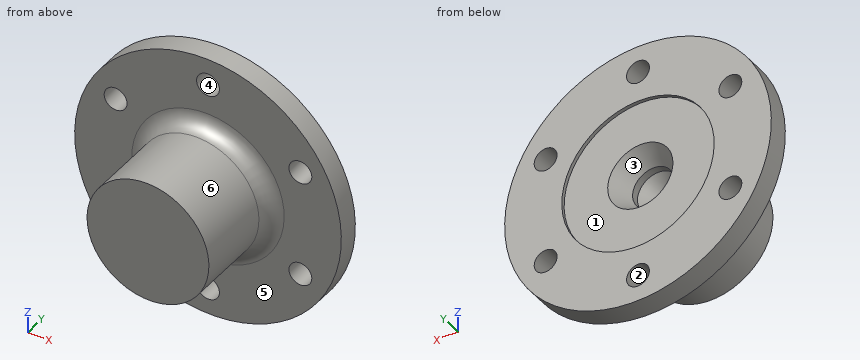
from build123d import *

# Parameters (mm, degrees)
F3_D            = 9.525
F3_COPIES_COUNT = 6


# Not quite as in the source:
# - a pattern or mirror of a feature is missing from the dataset's text; its kind, count and spacing are read off the source's solid


with BuildPart() as f1:
    # F0 (on Right) → F1 (revolve)
    with BuildSketch(Plane.YZ):
        with BuildLine():
            Line((8.89, 55.5625), (0, 55.5625))
            Line((0, 55.5625), (0, 31.75))
            ThreePointArc((0, 31.75), (-1.8598719395, 27.2598719395), (-6.35, 25.4))
            Line((-6.35, 25.4), (-38.1, 25.4))
            Line((-38.1, 25.4), (-38.1, 0))
            Line((-38.1, 0), (-16.51, 0))
            Line((-16.51, 0), (-13.335, 4.7625))
            Line((-13.335, 4.7625), (-9.0805, 4.7625))
            Line((-9.0805, 4.7625), (-3.81, 8.5725))
            Line((-3.81, 8.5725), (-0.7366, 8.5725))
            Line((-0.7366, 8.5725), (7.4295, 13.589))
            Line((7.4295, 13.589), (7.4295, 31.75))
            Line((7.4295, 31.75), (8.89, 31.75))
            Line((8.89, 31.75), (8.89, 55.5625))
        make_face()
    revolve(axis=Axis((0, -27.305, 0), (0, -1, 0)))

    # F3 (through all)
    with Locations(Plane(origin=(0, 8.89, 0), x_dir=(-1, 0, 0), z_dir=(0, 1, 0))):
        with Locations((0, 44.45)):
            f3 = Hole(F3_D / 2)

    # F3_copies: F3 ×6 about axis
    f3_copies_axis = Axis((0, 0, 0), (0, 1, 0))
    for i in range(1, F3_COPIES_COUNT):
        add(f3.rotate(f3_copies_axis, i * 360 / F3_COPIES_COUNT), mode=Mode.SUBTRACT)


solid = f1.part
Work out the finished part from the listing and answer in its coordinate system (mm). Face numbers are marked on the shaded views. A direction names the side the tool comes from. Give positions to 0.01 mm unless a question says otherwise; leave off trailing zeros. Order: outer loops, then holes, each group sorted by start corner. A loop starts at its lowest first (then second) coordinate and runs counter-clockwise, first axis right, second up. Notation, with made-up numbers: (87, 6.25) - (134, 6.25) arc R13 ccw to (134, 20.25) - close; hole circle Ø5 at (-33, 79). An arc over 180 degrees is marked (long way). Answer as CSV lines item,"result". Start each with the question number.
Q1. The part is cut by section C-C (x = -45.5). Write down the section's boundary in (y, z).
Q2. For the marked faces 1 and 2, determine the directions among +Z, -Z, +X, -X, +Y, -Y from which every point of the face is accessible in a straight line to the end or side of a thin tool.
Q3. The part is cut by section A-A (z = 44.45). Write down the section's boundary in (x, y).
Q4. Given pin 1 Ø1 at (y, z) = (0.5, -7.5) entering from +X; pin 2 Ø1.5 at (y, z) = (-31, -8) entering from +X; pin 3 Ø1.5 at (x, y) = (-7.5, -22.5) entering from -Z, each flat-ended and moving along its own axis, determine where each tip first touches the part or whether it passes through.
Q5. The part is cut by section B-B (y = -25). Write down the section's boundary in (x, z).
Q6. Find the intervals of material crossed by L1, parallel to Z at x = 0, y = -12.05; L2, parallel to X at y = 8.5, z = 0; L3, parallel to Y at x = -5.5, z = 19, in increasing order. Write a range as [from, to].
Q7. The mould has two halves that part along Z. Classify the marked faces 3, 4, 5 and 6: +Z half, -Z half, draft (parallel to the pull), parting line (faces both ways), or undercut.
Check result:
1,outline,"(0, -31.89) - (8.89, -31.89) - (8.89, 31.89) - (0, 31.89) - close"
2,face 1,"+Y"
2,face 2,"+Y, -Y"
3,outline,"(-33.34, 0) - (-4.76, 0) - (-4.76, 8.89) - (-33.34, 8.89) - close; (4.76, 0) - (33.34, 0) - (33.34, 8.89) - (4.76, 8.89) - close"
4,pin 1,"stops at x = 55.12"
4,pin 2,"stops at x = 24.34"
4,pin 3,"stops at z = -24.49"
5,outline,"circle Ø50.8 at (0, 0)"
6,L1,"z = [-25.4, -4.76], [4.76, 25.4]"
6,L2,"x = [-55.56, -31.75], [31.75, 55.56]"
6,L3,"y = [-38.1, 7.43]"
7,face 3,"undercut"
7,face 4,"undercut"
7,face 5,"draft"
7,face 6,"parting line"
